```python
from build123d import *

# Parameters (mm, degrees)
SKETCH1_R         = 5.188
BASENUT_DEPTH     = 12
SKETCH3_R         = 8.315
SKETCH3_R_2       = 5.188
EXTRUDE1_DEPTH    = 0.6
ENDCHAMFER3_SIZE  = 1.312
ENDCHAMFER3_SIZE2 = 0.757483553
LPATTERN10_COUNT  = 8
LPATTERN10_PITCH  = 1.5744


with BuildPart() as part:
    # Sketch1 → BaseNut (new body)
    with BuildSketch(Plane.XY):
        Polygon((5.196152423, -9), (10.392304845, 0), (5.196152423, 9), (-5.196152423, 9), (-10.392304845, 0), (-5.196152423, -9), align=None)
        Circle(SKETCH1_R, mode=Mode.SUBTRACT)
    extrude(amount=-BASENUT_DEPTH)

    # Sketch2 → Chamfer1 (revolve, cut)
    with BuildSketch(Plane(origin=(-16.706149795, 0, -15.04811501), x_dir=(0, 0, 1), z_dir=(0, 1, 0))):
        Polygon((3.04811501, 25.706149795), (3.04811501, 27.098454641), (3.851962587, 27.098454641), align=None)
    revolve(axis=Axis((0, 0, -38.770766557), (0, 0, 1)), mode=Mode.SUBTRACT)

    # Sketch6 → EndChamfer1 (revolve, cut)
    with BuildSketch(Plane(origin=(-9.197458863, 0, -10.252541137), x_dir=(0, 0, 1), z_dir=(0, 1, 0))):
        Polygon((-1.747458863, 14.385458863), (-1.747458863, 15.697458863), (-0.989975309, 14.385458863), align=None)
    revolve(axis=Axis((0, 0, 13.104863586), (0, 0, -1)), mode=Mode.SUBTRACT)

    # Sketch3 → Extrude1 (add)
    with BuildSketch(Plane(origin=(-18.48918612, 11.17895969, 0), x_dir=(1, 0, 0), z_dir=(0, 0, 1))):
        with Locations((18.48918612, -11.17895969)):
            Circle(SKETCH3_R)
        with Locations((18.48918612, -11.17895969)):
            Circle(SKETCH3_R_2, mode=Mode.SUBTRACT)
    extrude(amount=EXTRUDE1_DEPTH)

    # EndChamfer3
    endchamfer3_edges = [part.edges().sort_by_distance(p)[0] for p in [
        (-5.188, 0, 0.6),
    ]]
    endchamfer3_side = [part.faces().sort_by_distance(p)[0] for p in [
        (-8.079816285, 0, 0.6),
    ]]
    chamfer(endchamfer3_edges, length=ENDCHAMFER3_SIZE, length2=ENDCHAMFER3_SIZE2, reference=endchamfer3_side[0])

    # Sketch7 → Cut-Revolve10 (revolve, cut)
    with BuildSketch(Plane(origin=(0, 0, 0), x_dir=(1, 0, 0), z_dir=(0, 1, 0))):
        Polygon((3.876, 11.898516447), (5.188, 11.898516447), (6.32422533, 11.242516447), (5.188, 10.586516447), (3.876, 10.586516447), align=None)
    cut_revolve10 = revolve(axis=Axis((0, 0, -61.609777784), (0, 0, 1)), mode=Mode.SUBTRACT)

    # LPattern10: Cut-Revolve10 ×8
    with Locations(*[(0, 0, i * LPATTERN10_PITCH) for i in range(1, LPATTERN10_COUNT)]):
        add(cut_revolve10, mode=Mode.SUBTRACT)


solid = part.part
```
Verification items for the finished model (mm, model axes). Round coordinates to 2 decimals unless told otherwise and drop trailing zeros. Write each loop counter-clockwise with the first axis right and the second up, starting at its lowest first coordinate (ties: lowest second). Pieces come first, ordered by that corner, then holes.
1. Section check B-B on y = -6. State how many separate pieces and enclosed holes the cut face has, plus the area to 3 significant figures.
2. Gauge pin test, flat ends, axial feed: P1, Ø9.5, axis at x = 0, y = 0, coming from the +Z side; P2, Ø4, axis at y = -6, z = -3, coming from the -X side. Record the tip position at first contact, or that the pin passes through.
3. Scan lines: L1, parallel to Y at x = 0, z = -2.5; L2, parallel to Z at x = 6.5, y = -6; L3, parallel to X at y = -1.75, z = -1.75. Record each from-to range of solid material in increasing order.
4. Section check A-A on z = -7.75. Enter the section's corners in (x, y), plus the area to 3 significant figures.
Answer:
1. separate pieces: 1
1. enclosed holes: 8
1. area: 163 mm2
2. P1: passes through
2. P2: stops at x = -8.08
3. L1: y = -9 to -5.19, 5.19 to 9
3. L2: z = -12 to 0
3. L3: x = -9.38 to -5.99, 5.99 to 9.38
4. outline: (-10.39, 0) - (-5.2, -9) - (5.2, -9) - (10.39, 0) - (5.2, 9) - (-5.2, 9) - close; hole circle Ø11.46 at (0, 0)
4. area: 177 mm2
